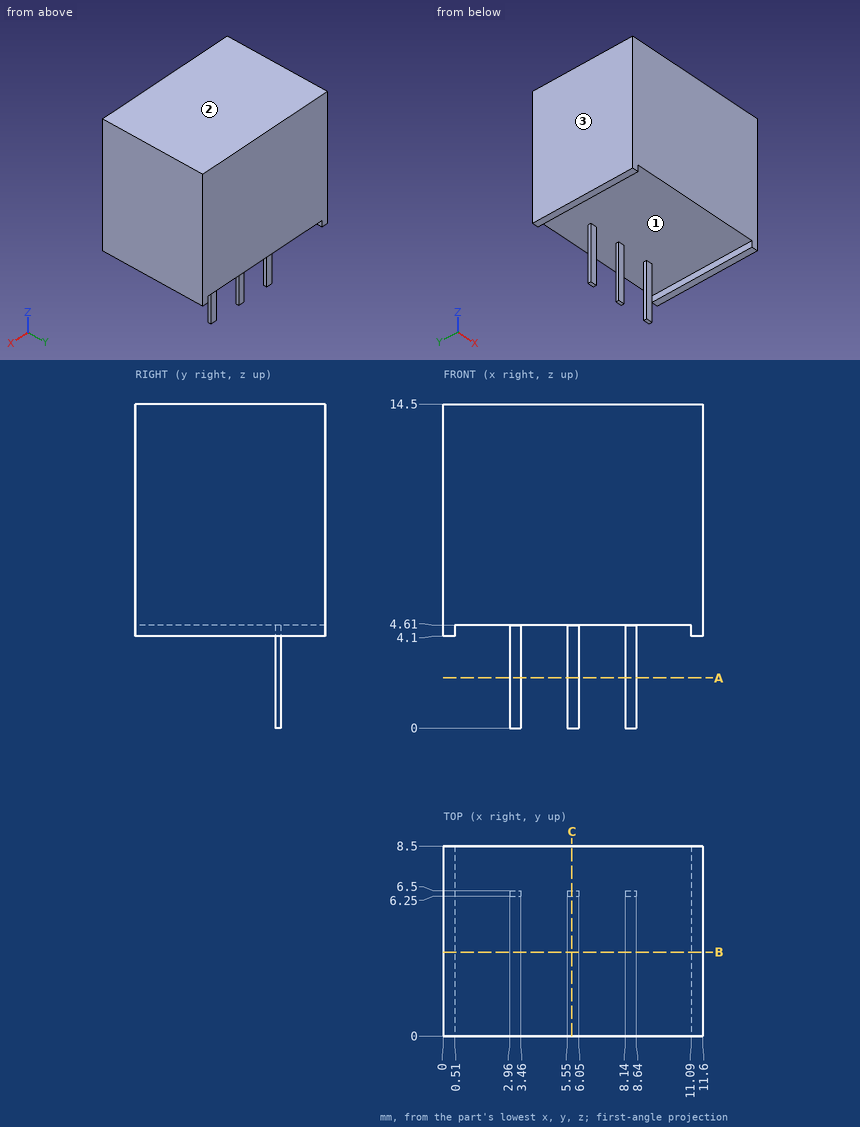
Geometry check sheet. Reference: drawing and pictorial views, mm from the part's lowest x, y, z. Give positions to 0.01 mm unless a question says otherwise; leave off trailing zeros. Loops run counter-clockwise (first coordinate to the right, second up) from the corner with the lowest first, then second, coordinate; pieces in that order, holes last. Notation, with made-up numbers: (-6, 17) -> (23, 17) arc R24 ccw to (23, 51) -> close; hole circle Ø10 at (-11.75, 28). An arc over 180 degrees is marked (long way). Answer in a Markdown table with one row per item. Add a question column.
1) Draft check along X on the marked faces 1, 2 and 3. Enter one of: pulls with the +X half, pulls with the -X half, needs draft (parallel to the pull), parting line crosses it, or undercut.
2) Cross-section at C-C on x = 5.75. Record the boundary of the cut face in (y, z).
3) Cross-section at A-A on z = 2.25. Record the boundary of the cut face in (x, y), and give its area (3 significant figures).
4) Material ranges on probe 1 along X at (y, z) = (6, 4.5); probe 2 along Z at (x, y) = (3, 3.75), recorded low to high. Write a range as from..to.
5) Cross-section at B-B on y = 3.75. Record the boundary of the cut face in (x, z), and give its area (3 significant figures).
Outcome:
| question | item | result |
|---|---|---|
| 1 | face 1 | undercut |
| 1 | face 2 | needs draft |
| 1 | face 3 | pulls with the -X half |
| 2 | outline | (0, 4.61) -> (6.25, 4.61) -> (6.25, 0) -> (6.5, 0) -> (6.5, 4.61) -> (8.5, 4.61) -> (8.5, 14.5) -> (0, 14.5) -> close |
| 3 | outline | (2.96, 6.25) -> (3.46, 6.25) -> (3.46, 6.5) -> (2.96, 6.5) -> close; (5.55, 6.25) -> (6.05, 6.25) -> (6.05, 6.5) -> (5.55, 6.5) -> close; (8.14, 6.25) -> (8.64, 6.25) -> (8.64, 6.5) -> (8.14, 6.5) -> close |
| 3 | area | 0.375 mm^2 |
| 4 | probe 1 | x = 0..0.51, 11.09..11.6 |
| 4 | probe 2 | z = 4.61..14.5 |
| 5 | outline | (0, 4.1) -> (0.51, 4.1) -> (0.51, 4.61) -> (11.09, 4.61) -> (11.09, 4.1) -> (11.6, 4.1) -> (11.6, 14.5) -> (0, 14.5) -> close |
| 5 | area | 115 mm^2 |
